Geometry check sheet. Reference: the model listing, model coordinates, mm. A direction names the side the tool comes from. Round coordinates to 2 decimals unless told otherwise and drop trailing zeros. Loops run counter-clockwise (first coordinate to the right, second up) from the corner with the lowest first, then second, coordinate; pieces in that order, holes last.
```python
from build123d import *

# Parameters (mm, degrees)
F0_W     = 80
F0_H     = 50
F1_DEPTH = 85
F3_DEPTH = 30
F5_W     = 25
F5_H     = 12.5
F6_DEPTH = 30
F7_DEPTH = 80
F9_DEPTH = 50


with BuildPart() as f1:
    # F0 (on Front) → F1 (new body)
    with BuildSketch(Plane.XZ):
        with Locations((40, 25)):
            Rectangle(F0_W, F0_H)
    extrude(amount=-F1_DEPTH)

    # F2 (on Right) → F3 (cut)
    with BuildSketch(Plane.YZ):
        Polygon((47.5, 10), (55, 10), (72.5, 10), (72.5, 22.5), (47.5, 22.5), align=None)
    extrude(amount=F3_DEPTH, mode=Mode.SUBTRACT)

    # F5 (on offset) → F6 (cut)
    with BuildSketch(Plane.YZ.offset(80)):
        with Locations((60, 16.25)):
            Rectangle(F5_W, F5_H)
    extrude(amount=-F6_DEPTH, mode=Mode.SUBTRACT)

    # F2 (on Right) → F7 (cut)
    with BuildSketch(Plane.YZ):
        Polygon((0, 30), (0, 0), (30, 50), (0, 50), align=None)
    extrude(amount=F7_DEPTH, mode=Mode.SUBTRACT)

    # F8 (on face) → F9 (cut)
    with BuildSketch(Plane(origin=(0, 85, 0), x_dir=(-1, 0, 0), z_dir=(0, 1, 0))):
        with BuildLine():
            ThreePointArc((-46.8738635424, 50), (-56.1206389452, 31.4821881801), (-40, 18.5))
            ThreePointArc((-40, 18.5), (-28.3327381104, 23.3327381104), (-23.5, 35))
            ThreePointArc((-23.5, 35), (-26.1135182921, 43.9115445224), (-33.1261364576, 50))
            Line((-33.1261364576, 50), (-46.8738635424, 50))
        make_face()
    extrude(amount=-F9_DEPTH, mode=Mode.SUBTRACT)


solid = f1.part
```
1) Scan lines: line 1 along Z through (x, y) = (64.5, 66); line 2 along X through (y, z) = (71.5, 34.5); line 3 along X through (y, z) = (64.5, 47.5). Record each from-to range of solid material in increasing order.
Report:
line 1: z = 0 to 10, 22.5 to 50
line 2: x = 0 to 23.51, 56.49 to 80
line 3: x = 0 to 29.23, 50.77 to 80
2) Mould release check, pull along Y, two halves, no side actions. Record for faces 1 (the face through (80, 51, 25)), 2 (the face through (50, 60, 16)), 3 (the face through (14, 60, 22.5)), 4 (the face through (40, 35, 34)): +Y half, -Y half, draft (parallel to the pull), parting line (faces both ways), or undercut.
Report:
face 1: draft
face 2: undercut
face 3: undercut
face 4: +Y half
3) Sectioned sample at A-A, the plane x = 63.5. Record the cut outline in (y, z).
Report:
outline: (0, 0) - (85, 0) - (85, 50) - (30, 50) - close; hole (47.5, 10) - (72.5, 10) - (72.5, 22.5) - (47.5, 22.5) - close
4) Sectioned sample at B-B, the plane y = 50.5. Record the cut outline in (x, z).
Report:
outline: (0, 0) - (80, 0) - (80, 10) - (50, 10) - (50, 21.88) arc R16.5 cw to (30, 21.88) - (30, 10) - (0, 10) - close; (0, 22.5) - (29.23, 22.5) arc R16.5 cw to (33.13, 50) - (0, 50) - close; (46.87, 50) arc R16.5 cw to (50.77, 22.5) - (80, 22.5) - (80, 50) - close
5) Sectioned sample at D-D, the plane x = 35. Record the cut outline in (y, z).
Report:
outline: (0, 0) - (85, 0) - (85, 19.28) - (35, 19.28) - (35, 50) - (30, 50) - close
6) Gauge pin test, flat ends, axial feed: pin 1 (4 mm diameter, centred on x = 12.5, z = 17.5, fed in from -Y); pin 2 (6 mm diameter, centred on y = 74, z = 42, fed in from -X); pin 3 (4 mm diameter, centred on x = 61.5, z = 18.5, fed in from -Y); pin 4 (1.5 mm diameter, centred on x = 33.5, y = 20.5, fed in from +Z). Record the tip position at first contact, or that the pin passes through.
Report:
pin 1: stops at y = 9.3
pin 2: stops at x = 0
pin 3: stops at y = 9.9
pin 4: stops at z = 35.42
7) Access from +Z, -Z, +X, -X, +Y, -Y to the whole of each face (thin tool, end or side, straight path). Record for faces 5 (the face through (65, 72.5, 16)), 6 (the face through (39, 85, 14)), 7 (the face through (39, 15, 25)), 8 (the face through (15, 47.5, 16)), 9 (the face through (66, 60, 22.5)).
Report:
face 5: +X
face 6: +Z, -Z, +X, -X, +Y
face 7: +Z, +X, -X, -Y
face 8: -X
face 9: +X, -X
8) Sectioned sample at C-C, the plane z = 43.5. Record the cut outline in (x, y), then the cut area to 3 significant figures.
Report:
outline: (0, 26.1) - (80, 26.1) - (80, 85) - (54.14, 85) - (54.14, 35) - (25.86, 35) - (25.86, 85) - (0, 85) - close
area: 3,300 mm2
